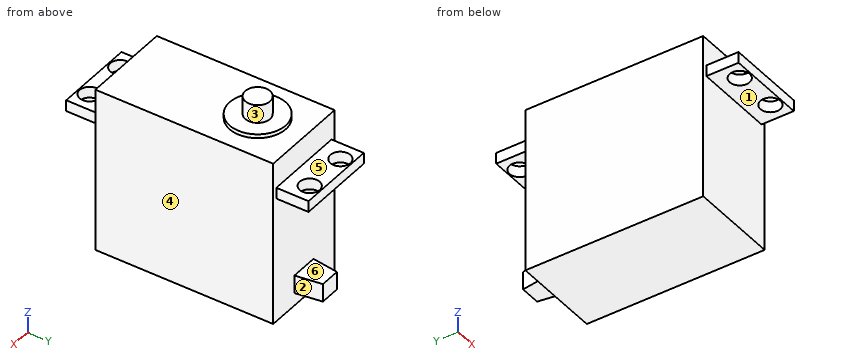
```python
from build123d import *

# Parameters (mm, degrees)
SKETCH1_W           = 20
SKETCH1_H           = 40
BOSS_EXTRUDE1_DEPTH = 8.7
SKETCH2_W           = 20
SKETCH2_H           = 40
BOSS_EXTRUDE2_DEPTH = 28.5
SKETCH3_R           = 2.25
BOSS_EXTRUDE3_DEPTH = 2.5
SKETCH4_R           = 2.794
BOSS_EXTRUDE4_DEPTH = 5
BOSS_EXTRUDE6_DEPTH = 6.9596
SKETCH10_R          = 6.30555
BOSS_EXTRUDE7_DEPTH = 0.889
CUT_EXTRUDE1_DEPTH  = 2.8956


with BuildPart() as part:
    # Sketch1 → Boss-Extrude1 (new body)
    with BuildSketch(Plane.XY):
        with Locations((10, 20)):
            Rectangle(SKETCH1_W, SKETCH1_H)
    extrude(amount=BOSS_EXTRUDE1_DEPTH)

    # Sketch2 → Boss-Extrude2 (add)
    with BuildSketch(Plane(origin=(0, 0, 0), x_dir=(-1, 0, 0), z_dir=(0, 0, -1))):
        with Locations((-10, 20)):
            Rectangle(SKETCH2_W, SKETCH2_H)
    extrude(amount=BOSS_EXTRUDE2_DEPTH)

    # Sketch3 → Boss-Extrude3 (add)
    with BuildSketch(Plane.XY):
        Polygon((19, 0), (19, -7.25), (1, -7.25), (1, 0), (0, 0), (0, 40), (1, 40), (1, 47.25), (19, 47.25), (19, 40), (20, 40), (20, 0), align=None)
        with Locations((5, -4.75)):
            Circle(SKETCH3_R, mode=Mode.SUBTRACT)
        with Locations((15, -4.75)):
            Circle(SKETCH3_R, mode=Mode.SUBTRACT)
        with Locations((5, 44.75)):
            Circle(SKETCH3_R, mode=Mode.SUBTRACT)
        with Locations((15, 44.75)):
            Circle(SKETCH3_R, mode=Mode.SUBTRACT)
    extrude(amount=BOSS_EXTRUDE3_DEPTH)

    # Sketch4 → Boss-Extrude4 (add)
    with BuildSketch(Plane.XY.offset(8.7)):
        with Locations((10, 29.6)):
            Circle(SKETCH4_R)
    extrude(amount=BOSS_EXTRUDE4_DEPTH)

    # Sketch9 → Boss-Extrude6 (add)
    with BuildSketch(Plane(origin=(0, 0, -28.5), x_dir=(-1, 0, 0), z_dir=(0, 0, -1))):
        Polygon((-13.1115, 40), (-6.8885, 40), (-7.714, 45.842), (-12.286, 45.842), align=None)
    extrude(amount=-BOSS_EXTRUDE6_DEPTH)

    # Sketch10 → Boss-Extrude7 (add)
    with BuildSketch(Plane.XY.offset(8.7)):
        with Locations((10, 29.6)):
            Circle(SKETCH10_R)
    extrude(amount=BOSS_EXTRUDE7_DEPTH)

    # Sketch11 → Cut-Extrude1 (cut)
    with BuildSketch(Plane(origin=(0, 0, -28.5), x_dir=(-1, 0, 0), z_dir=(0, 0, -1))):
        Polygon((-12.286, 45.842), (-7.714, 45.842), (-6.8885, 40), (-13.1115, 40), align=None)
    extrude(amount=-CUT_EXTRUDE1_DEPTH, mode=Mode.SUBTRACT)


solid = part.part
```
Work out the finished part from the listing and answer in its coordinate system (mm). Face numbers are marked on the shaded views. A direction names the side the tool comes from. Give positions to 0.01 mm unless a question says otherwise; leave off trailing zeros. Write each loop counter-clockwise with the first axis right and the second up, starting at its lowest first coordinate (ties: lowest second). Pieces come first, ordered by that corner, then holes. Notation, with made-up numbers: (81.5, 20.25) -> (119.5, 20.25) arc R17 cw to (119.5, 25.25) -> close; hole circle Ø8 at (-4, 72.25). An arc over 180 degrees is marked (long way). Write item = value, one per line.
Q1. Section B-B on z = -23.5 is taken. Determine the outline of the cut face in (x, y).
Computed values:
outline = (0, 0) -> (20, 0) -> (20, 40) -> (13.11, 40) -> (12.29, 45.84) -> (7.71, 45.84) -> (6.89, 40) -> (0, 40) -> close
Q2. Section C-C on y = 44.75 is taken. Determine the outline of the cut face in (x, z), and give its area (3 significant figures).
Computed values:
outline = (1, 0) -> (2.75, 0) -> (2.75, 2.5) -> (1, 2.5) -> close; (7.25, 0) -> (12.75, 0) -> (12.75, 2.5) -> (7.25, 2.5) -> close; (7.56, -25.6) -> (12.44, -25.6) -> (12.44, -21.54) -> (7.56, -21.54) -> close; (17.25, 0) -> (19, 0) -> (19, 2.5) -> (17.25, 2.5) -> close
area = 42.3 mm^2
Q3. A tool of negligible diameter and unlimited length cuts with its end or side. For the marked faces 1, 2 and 3, from which of +Z, -Z, +X, -X, +Y, -Y can it reach the whole face along a straight path? Write none if from no direction.
Computed values:
face_1 = -Z, +X, -X, -Y
face_2 = -Z, +X, +Y
face_3 = +Z
Q4. For a pull along Z with two mould halves and no side action, classify the marked faces 4, 5 and 6 as pulls with the +Z half, pulls with the -Z half, needs draft (parallel to the pull), parting line crosses it, or undercut.
Computed values:
face_4 = needs draft
face_5 = pulls with the +Z half
face_6 = undercut
Q5. Section A-A on x = 5.75 is taken. Determine the outline of the cut face in (y, z).
Computed values:
outline = (-7.25, 0) -> (-6.87, 0) -> (-6.87, 2.5) -> (-7.25, 2.5) -> close; (-2.63, 0) -> (0, 0) -> (0, -28.5) -> (40, -28.5) -> (40, 0) -> (42.63, 0) -> (42.63, 2.5) -> (40, 2.5) -> (40, 8.7) -> (34.26, 8.7) -> (34.26, 9.59) -> (24.94, 9.59) -> (24.94, 8.7) -> (0, 8.7) -> (0, 2.5) -> (-2.63, 2.5) -> close; (46.87, 0) -> (47.25, 0) -> (47.25, 2.5) -> (46.87, 2.5) -> close
Q6. Consider line 1 along Y through (x, z) = (5, 1.7); line 2 along Y through (x, z) = (13, 3.5); line 3 along Z through (x, y) = (10.5, 33.5). Determine where each line is inside the solid, lowest interval first.
Computed values:
line_1 = -7.25 to -7, -2.5 to 42.5, 47 to 47.25
line_2 = 0 to 40
line_3 = -28.5 to 9.59
Q7. Section D-D on y = 29.6 is taken. Determine the outline of the cut face in (x, z).
Computed values:
outline = (0, -28.5) -> (20, -28.5) -> (20, 8.7) -> (16.31, 8.7) -> (16.31, 9.59) -> (12.79, 9.59) -> (12.79, 13.7) -> (7.21, 13.7) -> (7.21, 9.59) -> (3.69, 9.59) -> (3.69, 8.7) -> (0, 8.7) -> close
Q8. Flat-ended cylindrical pins translate along their axes: pin 1 Ø1.5 at (x, z) = (11, -4) entering from +Y; pin 2 Ø3 at (x, y) = (10.5, 42.5) entering from +Z; pin 3 Ø1 at (x, z) = (12.5, -14) entering from -Y. Find the tip coordinate at first contact, or state that the pin passes through.
Computed values:
pin_1 = 40
pin_2 = 2.5
pin_3 = 0
